Geometry: see drawing. Coordinates: mm, zero at the bounding-box minimum. A direction names the side the tool comes from. Coordinates: 2 decimals unless noted, no trailing zeros. Write each loop counter-clockwise with the first axis right and the second up, starting at its lowest first coordinate (ties: lowest second). Pieces come first, ordered by that corner, then holes.
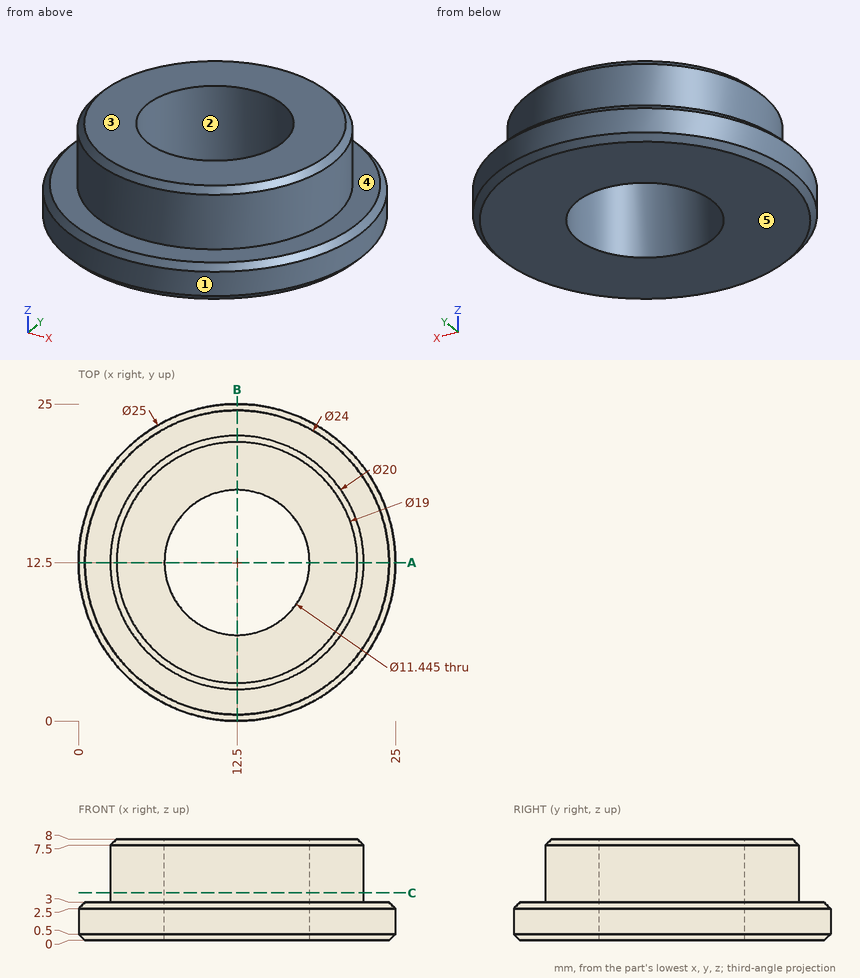
Item 1: Pin query (flat end, axial travel): pin 1 (7 mm diameter, centred on x = 12.5, y = 12.5, fed in from +Z); pin 2 (4 mm diameter, centred on x = 7, z = 4, fed in from +Y); pin 3 (3 mm diameter, centred on x = 9, z = 6, fed in from +Y). Return the tip coordinate at first contact, or that it passes through.
Derived:
pin 1: passes through
pin 2: stops at y = 24.28
pin 3: stops at y = 22.3
Item 2: Pull-direction query (X, two-part tool) for the marked faces 1, 2 and 3; classes: released by +X, released by -X, zero draft, split by the parting line, or undercut.
Derived:
face 1: split by the parting line
face 2: undercut
face 3: zero draft
Item 3: Section A-A, the plane y = 12.5. Output: boundary loops of the cut face in (x, z), plus the area to 3 significant figures.
Derived:
outline: (0, 0.5) - (0.5, 0) - (6.78, 0) - (6.78, 8) - (3, 8) - (2.5, 7.5) - (2.5, 3) - (0.5, 3) - (0, 2.5) - close; (18.22, 0) - (24.5, 0) - (25, 0.5) - (25, 2.5) - (24.5, 3) - (22.5, 3) - (22.5, 7.5) - (22, 8) - (18.22, 8) - close
area: 82.7 mm2
Item 4: Material intervals for probe 1 along Y at (x, z) = (12.5, 3.5); probe 2 along Y at (x, z) = (12.5, 2.5); probe 3 along Z at (x, y) = (9.25, 23.25), sorted ascending.
Derived:
probe 1: y = 2.5 to 6.78, 18.22 to 22.5
probe 2: y = 0 to 6.78, 18.22 to 25
probe 3: z = 0 to 3
Item 5: Set-up query: the marked faces 4 and 5. Return all of +Z, -Z, +X, -X, +Y, -Y with unobstructed straight access to the full face (end or side cutting, diameter ignored); none if empty.
Derived:
face 4: +Z
face 5: -Z, +X, -X, +Y, -Y
Item 6: Section C-C, the plane z = 3.75. Output: boundary loops of the cut face in (x, y) (1 decimal).
Derived:
outline: circle Ø20 at (12.5, 12.5); hole circle Ø11.4 at (12.5, 12.5)
